Here's how the part is built. I have some questions about the finished solid (model axes, mm). Round coordinates to 2 decimals unless told otherwise and drop trailing zeros. Write each loop counter-clockwise with the first axis right and the second up, starting at its lowest first coordinate (ties: lowest second). Pieces come first, ordered by that corner, then holes. Notation, with made-up numbers: (8, -26) -> (59, -26) arc R12 ccw to (59, -8) -> close; hole circle Ø11 at (-18, 40). An arc over 180 degrees is marked (long way). Put each result on its own line as item: value. Start each with the question number.
1. I need wall thicknesses on probe 1 along Y at (x, z) = (10.25, 0.75); probe 2 along Y at (x, z) = (10, 1.3); probe 3 along X at (y, z) = (8.5, 1.05). Which ranges of each line are inside material? Lowest first, please. Write a range as from..to.
2. We'd pull the mould along X, two halves only. Please class faces 1 (the face through (7.606, 11.285, 1.014)), 2 (the face through (9, 35, 2)): +X half, -X half, draft (parallel to the pull), parting line (faces both ways), or undercut.
3. Suppose I cut it at B-B (z = 1.15). Count the separate pieces of the cut face and the enclosed holes in it, then the cut area to 3 significant figures.
4. Suppose I cut it at A-A (x = 10.25). Please give me the cut outline in (y, z).
```python
from build123d import *

# Parameters (mm, degrees)
SKETCH022_W         = 19.05
SKETCH022_H         = 69.85
PAD009_DEPTH        = 2
SKETCH023_R         = 2.6035
POCKET011_DEPTH     = 2.001
LINEARPATTERN_COUNT = 2
LINEARPATTERN_PITCH = 50.8
FILLET008_R         = 0.5


with BuildPart() as part:
    # Sketch022 → Pad009 (new body)
    with BuildSketch(Plane.XY):
        with Locations((9.525, 34.925)):
            Rectangle(SKETCH022_W, SKETCH022_H)
    extrude(amount=PAD009_DEPTH)

    # Sketch023 (on Face6 of Pad009) → Pocket011 (cut, through all)
    with BuildSketch(Plane.XY.offset(2)):
        with Locations((9.525, 9.525)):
            Circle(SKETCH023_R)
    pocket011 = extrude(amount=-POCKET011_DEPTH, mode=Mode.SUBTRACT)

    # LinearPattern: Pocket011 ×2
    with Locations(*[(0, i * LINEARPATTERN_PITCH, 0) for i in range(1, LINEARPATTERN_COUNT)]):
        add(pocket011, mode=Mode.SUBTRACT)

    # Fillet008
    fillet008_edges = [part.edges().sort_by_distance(p)[0] for p in [
        (0, 0, 1),
        (19.05, 0, 1),
        (9.525, 0, 0),
        (9.525, 0, 2),
        (19.05, 69.85, 1),
        (19.05, 34.925, 0),
        (19.05, 34.925, 2),
        (0, 69.85, 1),
        (0, 34.925, 0),
        (0, 34.925, 2),
        (9.525, 69.85, 0),
        (9.525, 69.85, 2),
    ]]
    fillet(fillet008_edges, radius=FILLET008_R)


solid = part.part
```
Verdict:
1. probe 1: y = 0..7.02, 12.03..57.82, 62.83..69.85
1. probe 2: y = 0..6.97, 12.08..57.77, 62.88..69.85
1. probe 3: x = 0..7.13, 11.92..19.05
2. face 1: undercut
2. face 2: draft
3. separate pieces: 1
3. enclosed holes: 2
3. area: 1,290 mm^2
4. outline: (0, 0.5) arc R0.5 ccw to (0.5, 0) -> (7.02, 0) -> (7.02, 2) -> (0.5, 2) arc R0.5 ccw to (0, 1.5) -> close; (12.03, 0) -> (57.82, 0) -> (57.82, 2) -> (12.03, 2) -> close; (62.83, 0) -> (69.35, 0) arc R0.5 ccw to (69.85, 0.5) -> (69.85, 1.5) arc R0.5 ccw to (69.35, 2) -> (62.83, 2) -> close
